```python
from build123d import *

# Parameters (mm, degrees)
SKETCH1_R             = 80
SKETCH1_R_2           = 6
BOSS_EXTRUDE1_DEPTH   = 13
SKETCH2_R             = 65
CUT_EXTRUDE1_DEPTH    = 8
SKETCH3_R             = 13
SKETCH3_R_2           = 6
BOSS_EXTRUDE3_DEPTH   = 18
CHAMFER1_SIZE         = 1
CHAMFER1_SIZE2        = 1.732050808
CHAMFER1_PART_2_SIZE  = 1
CHAMFER1_PART_2_SIZE2 = 1.732050808
CHAMFER1_PART_3_SIZE  = 1
CHAMFER1_PART_3_SIZE2 = 1.732050808
CHAMFER1_PART_4_SIZE  = 1
CHAMFER1_PART_4_SIZE2 = 1.732050808
CUT_EXTRUDE2_DEPTH    = 24
CIRPATTERN1_COUNT     = 10


with BuildPart() as part:
    # Sketch1 → Boss-Extrude1 (new body, symmetric)
    with BuildSketch(Plane.XY):
        Circle(SKETCH1_R)
        Circle(SKETCH1_R_2, mode=Mode.SUBTRACT)
    extrude(amount=BOSS_EXTRUDE1_DEPTH, both=True)

    # Sketch2 → Cut-Extrude1 (cut)
    with BuildSketch(Plane.XY.offset(13)):
        Circle(SKETCH2_R)
    cut_extrude1 = extrude(amount=-CUT_EXTRUDE1_DEPTH, mode=Mode.SUBTRACT)

    # Mirror1: Cut-Extrude1 across plane
    add(cut_extrude1.mirror(Plane.XY), mode=Mode.SUBTRACT)

    # Sketch3 → Boss-Extrude3 (add, symmetric)
    with BuildSketch(Plane.XY):
        Circle(SKETCH3_R)
        Circle(SKETCH3_R_2, mode=Mode.SUBTRACT)
    extrude(amount=BOSS_EXTRUDE3_DEPTH, both=True)

    # Chamfer1
    chamfer1_edges = [part.edges().sort_by_distance(p)[0] for p in [
        (-65, 0, 13),
    ]]
    chamfer1_side = [part.faces().sort_by_distance(p)[0] for p in [
        (-77.7372583, 0, 13),
    ]]
    chamfer(chamfer1_edges, length=CHAMFER1_SIZE, length2=CHAMFER1_SIZE2, reference=chamfer1_side[0])

    # Chamfer1 part 2
    chamfer1_part_2_edges = [part.edges().sort_by_distance(p)[0] for p in [
        (-65, 0, -13),
    ]]
    chamfer1_part_2_side = [part.faces().sort_by_distance(p)[0] for p in [
        (-65, 0, -9),
    ]]
    chamfer(chamfer1_part_2_edges, length=CHAMFER1_PART_2_SIZE, length2=CHAMFER1_PART_2_SIZE2, reference=chamfer1_part_2_side[0])

    # Chamfer1 part 3
    chamfer1_part_3_edges = [part.edges().sort_by_distance(p)[0] for p in [
        (-80, 0, -13),
    ]]
    chamfer1_part_3_side = [part.faces().sort_by_distance(p)[0] for p in [
        (-77.7372583, 0, -13),
    ]]
    chamfer(chamfer1_part_3_edges, length=CHAMFER1_PART_3_SIZE, length2=CHAMFER1_PART_3_SIZE2, reference=chamfer1_part_3_side[0])

    # Chamfer1 part 4
    chamfer1_part_4_edges = [part.edges().sort_by_distance(p)[0] for p in [
        (-80, 0, 13),
    ]]
    chamfer1_part_4_side = [part.faces().sort_by_distance(p)[0] for p in [
        (-80, 0, 0),
    ]]
    chamfer(chamfer1_part_4_edges, length=CHAMFER1_PART_4_SIZE, length2=CHAMFER1_PART_4_SIZE2, reference=chamfer1_part_4_side[0])

    # Sketch4 → Cut-Extrude2 (cut, through all)
    with BuildSketch(Plane.XY.offset(5)):
        with BuildLine():
            Line((0, 54.772255751), (0, 19.397164741))
            ThreePointArc((0, 19.397164741), (-0.515032591, 18.057436487), (-1.794871795, 17.407711947))
            ThreePointArc((-1.794871795, 17.407711947), (-4.529333289, 16.90370196), (-7.149451403, 15.972956666))
            ThreePointArc((-7.149451403, 15.972956666), (-8.582686936, 15.895715021), (-9.698582371, 16.798437427))
            Line((-9.698582371, 16.798437427), (-27.386127875, 47.434164903))
            ThreePointArc((-27.386127875, 47.434164903), (-27.821744262, 51.446675992), (-25.152000934, 54.473634439))
            ThreePointArc((-25.152000934, 54.473634439), (-15.529142706, 57.955549577), (-5.454545455, 59.751551728))
            ThreePointArc((-5.454545455, 59.751551728), (-1.629000688, 58.46500048), (0, 54.772255751))
        make_face()
    cut_extrude2 = extrude(amount=-CUT_EXTRUDE2_DEPTH, mode=Mode.SUBTRACT)

    # CirPattern1: Cut-Extrude2 ×10 about axis
    cirpattern1_axis = Axis((0, 0, 0), (0, 0, 1))
    for i in range(1, CIRPATTERN1_COUNT):
        add(cut_extrude2.rotate(cirpattern1_axis, i * 360 / CIRPATTERN1_COUNT), mode=Mode.SUBTRACT)


solid = part.part
```
Build history of the part. All positions in model axes, mm. A direction names the side the tool comes from. Round coordinates to 2 decimals unless told otherwise and drop trailing zeros. Write each loop counter-clockwise with the first axis right and the second up, starting at its lowest first coordinate (ties: lowest second). Pieces come first, ordered by that corner, then holes.
1) Mould opens along Y. For faces 4 (the flat face through (-41, -52, 13)), 5 (the cylindrical face through (7.685, 57.94, 0.07)) say: +Y half, -Y half, draft (parallel to the pull), parting line (faces both ways), or undercut.
2) Drill centre lines: probe 1 along Y at (x, z) = (0, -9); probe 2 along X at (y, z) = (-10, -7); probe 3 along X at (y, z) = (4, -10.5). Where is each one in solid material? Low to high.
3) Band-saw the part on B-B, the plane y = 0. Give the number of separate pieces and of enclosed holes in the cut face, and give its area (3 significant figures).
4) Band-saw the part on A-A, the plane z = 8. List the corners of the cut face in (x, y).
5) Pin check, flat tips, straight feed: pin 1 (9.5 mm diameter, centred on x = 0, y = 0, fed in from +Z); pin 2 (4 mm diameter, centred on x = -43.5, z = -10, fed in from -Y); pin 3 (2 mm diameter, centred on y = -56, z = 8.5, fed in from +X); pin 4 (6 mm diameter, centred on x = -39, z = -4.5, fed in from -Y). Stop position of each tip, or through.
6) 3-axis set-ups, long thin cutter, end or side, ignore diameter. For faces 1 (the flat face through (21.94, -30.2, 0.07)), 2 (the cylindrical face through (-10.316, -7.91, 11.591)), 3 (the cylindrical face through (-10.316, -7.91, -11.409)): which of +Z, -Z, +X, -X, +Y, -Y reach the whole face in a straight line?
Ans:
1. face 4: draft
1. face 5: undercut
2. probe 1: y = -80 to -65, -13 to -6, 6 to 13, 65 to 80
2. probe 2: x = -79.37 to -64.23, -8.31 to 8.31, 64.23 to 79.37
2. probe 3: x = -79.9 to -64.88, -12.37 to -4.47, 4.47 to 12.37, 64.88 to 79.9
3. separate pieces: 4
3. enclosed holes: 0
3. area: 1,470 mm2
4. outline: circle Ø160 at (0, 0); circle Ø26 at (0, 0); hole circle Ø130 at (0, 0); hole circle Ø12 at (0, 0)
5. pin 1: passes through
5. pin 2: stops at y = -68.39
5. pin 3: stops at x = 58.09
5. pin 4: stops at y = -71.44
6. face 1: +Z, -Z
6. face 2: +Z
6. face 3: -Z
